For this review, take the finished solid that the model builds, in its own axes (mm). A direction names the side the tool comes from. Round coordinates to 2 decimals unless told otherwise and drop trailing zeros. Write each loop counter-clockwise with the first axis right and the second up, starting at its lowest first coordinate (ties: lowest second). Pieces come first, ordered by that corner, then holes. Notation, with made-up numbers: (29, 85) -> (66, 85) arc R34 ccw to (66, 117) -> close; hole circle Ø7 at (4.25, 9.25). An arc over 180 degrees is marked (long way). Answer as CSV lines item,"result". Start each with the question number.
Item 1: Mouldability with a two-part tool opening along X and no side actions: class faces 1 (the cylindrical face through (244.237, 61.17, -23.979)), 2 (the flat face through (3, 14, -19.5)), 3 (the flat face through (227.71, 37.876, -23.979)) as +X half, -X half, draft (parallel to the pull), parting line (faces both ways), or undercut.
Item 2: Machinability: for faces 4 (the flat face through (-191.76, 60.026, 0.315)), 5 (the flat face through (180, 2, -2)), 6 (the flat face through (191.76, 60.026, 0.315)), 7 (the flat face through (2, 12, -22.5)), which of the approach directions +Z, -Z, +X, -X, +Y, -Y give a long, thin tool a straight path to every point of the face, cutting with its end or side? Answer none if there is none.
Item 3: Take a section at C-C on x = 58. Give the boundary of the cut face in (y, z), then the cut area to 3 significant figures.
Item 4: Take a section at D-D on y = 65. Count the separate pieces of the cut face and the enclosed holes in it, then the cut area to 3 significant figures.
Item 5: Wall thickness on probe 1 along Z at (x, y) = (200, 14); probe 2 along Z at (x, y) = (87.5, 20.5); probe 3 along Y at (x, z) = (66, -0.5): over which ranges is each line inside the solid? List them lowest first. Write a range as from..to.
Item 6: For pin 1 Ø0.9 at (y, z) = (6.5, -24) entering from +X; pin 2 Ø10 at (x, z) = (-57.5, 2) entering from +Y; pin 3 Ø2 at (y, z) = (65.5, -4.5) entering from +X, all flat-tipped, find the tip position at first contact; note any pin that passes through.
Item 7: Take a section at A-A on z = 7.5. Give the boundary of the cut face in (x, y), then the cut area to 3 significant figures.
Item 8: Take a section at B-B on x = -235. Give the boundary of the cut face in (y, z), then the cut area to 3 significant figures.
```python
from build123d import *

# Parameters (mm, degrees)
EXTRUDE_1_DEPTH          = 180
SKETCH_2_R               = 10
EXTRUDE_2_DEPTH          = 3
EXTRUDE_3_DEPTH          = 22.5
MIRROR_2_COPY_1_SKETCH_R = 10
MIRROR_2_COPY_1_DEPTH    = 3


with BuildPart() as part:
    # 스케치1 → 보스-돌출1 (new, symmetric)
    with BuildSketch(Plane(origin=(0, 0, 0), x_dir=(0, 0, -1), z_dir=(1, 0, 0))):
        Polygon((22.5, 0), (22.5, 25), (19.5, 25), (19.5, 3), (-19.5, 3), (-19.5, 25), (-22.5, 25), (-22.5, 0), align=None)
    extrude(amount=EXTRUDE_1_DEPTH, both=True)

    # 스케치2 → 보스-돌출2 (add)
    with BuildSketch(Plane.XY.offset(22.5)):
        with BuildLine():
            Line((155, 0), (155, 36.807573628))
            ThreePointArc((155, 36.807573628), (156.359363128, 41.841398659), (160.067878888, 45.506664462))
            Line((160.067878888, 45.506664462), (225.135757776, 82.398181668))
            ThreePointArc((225.135757776, 82.398181668), (252.398181668, 74.864242224), (244.864242224, 47.601818332))
            Line((244.864242224, 47.601818332), (210.067878888, 27.873333884))
            ThreePointArc((210.067878888, 27.873333884), (206.359363128, 24.208068081), (205, 19.17424305))
            Line((205, 19.17424305), (205, 0))
            Line((205, 0), (155, 0))
        make_face()
        with Locations((235, 65)):
            Circle(SKETCH_2_R, mode=Mode.SUBTRACT)
    extrude_2 = extrude(amount=EXTRUDE_2_DEPTH)

    # 대칭 복사1: 보스-돌출2 across plane
    add(extrude_2.mirror(Plane.XY))

    # 스케치4 → 보스-돌출3 (add, symmetric)
    with BuildSketch(Plane.XY):
        Polygon((170, 51.137876408), (210, 73.816665289), (211.479636334, 71.206938039), (171.479636334, 48.528149158), align=None)
    extrude_3 = extrude(amount=EXTRUDE_3_DEPTH, both=True)

    # 대칭 복사2: 보스-돌출2, 보스-돌출3 across plane
    add(extrude_2.mirror(Plane(origin=(0, 0, 0), x_dir=(0, 0, 1), z_dir=(1, 0, 0))))
    add(extrude_3.mirror(Plane(origin=(0, 0, 0), x_dir=(0, 0, 1), z_dir=(1, 0, 0))))

    # 대칭 복사2 copy 1 sketch → 대칭 복사2 copy 1 (add)
    with BuildSketch(Plane(origin=(0, 0, -22.5), x_dir=(-1, 0, 0), z_dir=(0, 0, -1))):
        with BuildLine():
            Line((155, 0), (155, 36.807573628))
            ThreePointArc((155, 36.807573628), (156.359363128, 41.841398659), (160.067878888, 45.506664462))
            Line((160.067878888, 45.506664462), (225.135757776, 82.398181668))
            ThreePointArc((225.135757776, 82.398181668), (252.398181668, 74.864242224), (244.864242224, 47.601818332))
            Line((244.864242224, 47.601818332), (210.067878888, 27.873333884))
            ThreePointArc((210.067878888, 27.873333884), (206.359363128, 24.208068081), (205, 19.17424305))
            Line((205, 19.17424305), (205, 0))
            Line((205, 0), (155, 0))
        make_face()
        with Locations((235, 65)):
            Circle(MIRROR_2_COPY_1_SKETCH_R, mode=Mode.SUBTRACT)
    extrude(amount=MIRROR_2_COPY_1_DEPTH)


solid = part.part
```
Output values:
1,face 1,"undercut"
1,face 2,"draft"
1,face 3,"+X half"
2,face 4,"-X"
2,face 5,"+X, -Y"
2,face 6,"+X"
2,face 7,"-Z, +Y, -Y"
3,outline,"(0, -22.5) -> (25, -22.5) -> (25, -19.5) -> (3, -19.5) -> (3, 19.5) -> (25, 19.5) -> (25, 22.5) -> (0, 22.5) -> close"
3,area,"267 mm^2"
4,separate pieces,"6"
4,enclosed holes,"0"
4,area,"1,030 mm^2"
5,probe 1,"z = -25.5..-22.5, 22.5..25.5"
5,probe 2,"z = -22.5..-19.5, 19.5..22.5"
5,probe 3,"y = 0..3"
6,pin 1,"stops at x = 205"
6,pin 2,"stops at y = 3"
6,pin 3,"stops at x = 203.18"
7,outline,"(-211.48, 71.21) -> (-171.48, 48.53) -> (-170, 51.14) -> (-210, 73.82) -> close; (-180, 0) -> (180, 0) -> (180, 3) -> (-180, 3) -> close; (170, 51.14) -> (171.48, 48.53) -> (211.48, 71.21) -> (210, 73.82) -> close"
7,area,"1,360 mm^2"
8,outline,"(42.01, -25.5) -> (55, -25.5) -> (55, -22.5) -> (42.01, -22.5) -> close; (42.01, 22.5) -> (55, 22.5) -> (55, 25.5) -> (42.01, 25.5) -> close; (75, -25.5) -> (85, -25.5) -> (85, -22.5) -> (75, -22.5) -> close; (75, 22.5) -> (85, 22.5) -> (85, 25.5) -> (75, 25.5) -> close"
8,area,"138 mm^2"
